Source: CAD feature listing. Evaluate the final solid. Frame: model axes, mm. Coordinates: 2 decimals unless noted, no trailing zeros. Loops run counter-clockwise (first coordinate to the right, second up) from the corner with the lowest first, then second, coordinate; pieces in that order, holes last.
Item 1: Line query: probe 1 along Z at (x, y) = (-8.5, 0.75); probe 2 along X at (y, z) = (1.75, -123); probe 3 along Z at (x, y) = (-16.5, 1.5). Output: solid intervals per line, ascending.
Item 2: Pin query (flat end, axial travel): pin 1 Ø6 at (x, y) = (-29, 2.5) entering from +Z; pin 2 Ø3 at (x, y) = (-30, 5) entering from -Z; pin 3 Ø5.5 at (y, z) = (3, -148) entering from -X. Return the tip coordinate at first contact, or that it passes through.
Item 3: Section query B-B, the plane x = -44. Return the cut outline in (y, z), then the cut area to 3 significant figures.
Item 4: Section query C-C, the plane z = -16.5. Return the cut outline in (x, y).
Item 5: Section query A-A, the plane z = -123. Return the cut outline in (x, y), then the cut area to 3 significant figures.
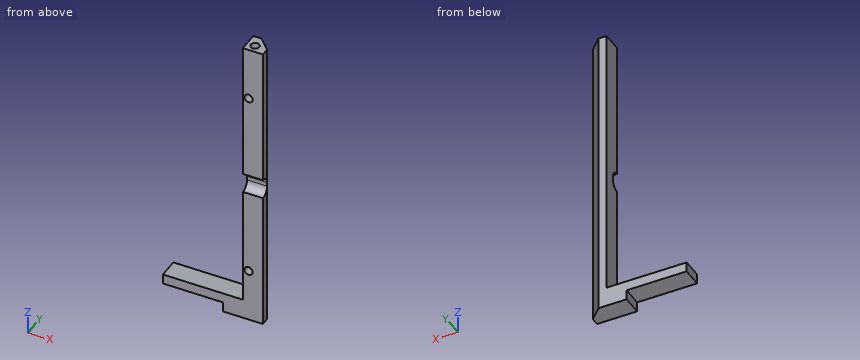
```python
from build123d import *

# Parameters (mm, degrees)
DODANIE_WYCI_GNI_CIE1_DEPTH = 10
SZKIC2_R                    = 2.1
WYTNIJ_WYCI_GNI_CIE1_DEPTH  = 4
SZKIC3_R                    = 2.1
WYTNIJ_WYCI_GNI_CIE2_DEPTH  = 4
SFAZOWANIE1_SIZE            = 6
SZKIC4_W                    = 10
SZKIC4_H                    = 10
WYTNIJ_WYCI_GNI_CIE3_DEPTH  = 4
ZAOKR_GLENIE1_R             = 4


with BuildPart() as part:
    # Szkic1 → Dodanie-wyciągnięcie1 (new body)
    with BuildSketch(Plane(origin=(0, 0, 0), x_dir=(1, 0, 0), z_dir=(0, 1, 0))):
        Polygon((0, 0), (0, 150), (-20, 150), (-20, 145), (-50, 145), (-50, 140), (-10, 140), (-10, 0), align=None)
    extrude(amount=DODANIE_WYCI_GNI_CIE1_DEPTH)

    # Szkic2 → Wytnij-wyciągnięcie1 (cut)
    with BuildSketch(Plane.XZ):
        with Locations(Location((-7.2, -123, 0), (0, 0, 270))):
            Circle(SZKIC2_R)
        with Locations(Location((-7.2, -27, 0), (0, 0, 270))):
            Circle(SZKIC2_R)
    extrude(amount=-WYTNIJ_WYCI_GNI_CIE1_DEPTH, mode=Mode.SUBTRACT)

    # Szkic3 → Wytnij-wyciągnięcie2 (cut)
    with BuildSketch(Plane.XY):
        with Locations((-6, 4)):
            Circle(SZKIC3_R)
    extrude(amount=-WYTNIJ_WYCI_GNI_CIE2_DEPTH, mode=Mode.SUBTRACT)

    # Sfazowanie1
    sfazowanie1_edges = [part.edges().sort_by_distance(p)[0] for p in [
        (0, 10, -75),
    ]]
    chamfer(sfazowanie1_edges, length=SFAZOWANIE1_SIZE)

    # Szkic4 → Wytnij-wyciągnięcie3 (cut)
    with BuildSketch(Plane.XZ):
        with Locations((-5, -75)):
            Rectangle(SZKIC4_W, SZKIC4_H)
    extrude(amount=-WYTNIJ_WYCI_GNI_CIE3_DEPTH, mode=Mode.SUBTRACT)

    # Zaokrąglenie1
    zaokr_glenie1_edges = [part.edges().sort_by_distance(p)[0] for p in [
        (-5, 4, -80),
        (-5, 4, -70),
    ]]
    fillet(zaokr_glenie1_edges, radius=ZAOKR_GLENIE1_R - 0.0001)  # a hair under: the kernel refuses the full size


solid = part.part
```
Verdict:
1. probe 1: z = -150 to -124.65, -121.35 to -79.93, -70.07 to -28.65, -25.35 to 0
1. probe 2: x = -10 to -9.3, -5.1 to 0
1. probe 3: z = -150 to -140
2. pin 1: stops at z = -140
2. pin 2: stops at z = -145
2. pin 3: stops at x = -20
3. outline: (0, -145) - (10, -145) - (10, -140) - (0, -140) - close
3. area: 50.0 mm2
4. outline: (-10, 0) - (0, 0) - (0, 4) - (-6, 10) - (-10, 10) - close
5. outline: (-10, 0) - (-9.3, 0) - (-9.3, 4) - (-5.1, 4) - (-5.1, 0) - (0, 0) - (0, 4) - (-6, 10) - (-10, 10) - close
5. area: 65.2 mm2
